```python
from build123d import *

# Parameters (mm, degrees)
F0_R     = 12.7
F1_DEPTH = 30.1625


with BuildPart() as f1:
    # F0 (on Front) → F1 (new body, symmetric)
    with BuildSketch(Plane.XZ):
        with BuildLine():
            Line((117.2464, 0), (22.352, 0))
            ThreePointArc((22.352, 0), (-15.805251, 15.805251), (0, -22.352))
            Line((0, -22.352), (194.2084, -22.352))
            Line((194.2084, -22.352), (194.2084, -7.874))
            ThreePointArc((194.2084, -7.874), (191.902159, -2.306241), (186.3344, 0))
            Line((186.3344, 0), (150.0886, 0))
            Line((150.0886, 0), (150.0886, 29.718))
            ThreePointArc((150.0886, 29.718), (148.600702, 33.310102), (145.0086, 34.798))
            Line((145.0086, 34.798), (131.0386, 34.798))
            ThreePointArc((131.0386, 34.798), (127.464415, 16.082358), (117.2464, 0))
        make_face()
        Circle(F0_R, mode=Mode.SUBTRACT)
    extrude(amount=F1_DEPTH, both=True)


solid = f1.part
```
Geometry check sheet. Reference: the model listing, model coordinates, mm. A direction names the side the tool comes from. Round coordinates to 2 decimals unless told otherwise and drop trailing zeros. Loops run counter-clockwise (first coordinate to the right, second up) from the corner with the lowest first, then second, coordinate; pieces in that order, holes last. Notation, with made-up numbers: (88.5, 2.25) - (117.5, 2.25) arc R17 ccw to (117.5, 22.25) - close; hole circle Ø4 at (-8.5, 86.5). An arc over 180 degrees is marked (long way). Use a Markdown table: item, result.
Q1. Go/stop test with flat-tipped pins: P1, Ø4, axis at x = 165.5, y = -19, coming from the +Z side; P2, Ø2, axis at y = 7, z = 29, coming from the -X side; P3, Ø12, axis at y = -2.5, z = 28.5, coming from the +X side. Record where each tip stops, or that it passes through.
Solutions:
| item | result |
|---|---|
| P1 | stops at z = 0 |
| P2 | stops at x = 130.58 |
| P3 | stops at x = 150.09 |
Q2. Cross-section at C-C on x = 93. Record the cut outline in (y, z).
Solutions:
| item | result |
|---|---|
| outline | (-30.16, -22.35) - (30.16, -22.35) - (30.16, 0) - (-30.16, 0) - close |
Q3. Material ranges on line 1 (Z direction, x = 0, y = -3); line 2 (X direction, y = 2, z = 4); line 3 (Z direction, x = 70, y = 26), recorded low to high.
Solutions:
| item | result |
|---|---|
| line 1 | z = -22.35 to -12.7, 12.7 to 22.35 |
| line 2 | x = -21.99 to -12.05, 12.05 to 21.99, 120.64 to 150.09 |
| line 3 | z = -22.35 to 0 |
Q4. Draft check along X on faces 4 (the cylindrical face through (191.963, -0.422, -2.368)), 5 (the flat face through (84, 30.162, -6)), 6 (the cylindrical face through (127.56, -0.42, 16.33)). Enter one of: released by +X, released by -X, zero draft, split by the parting line, or undercut.
Solutions:
| item | result |
|---|---|
| face 4 | released by +X |
| face 5 | zero draft |
| face 6 | undercut |
Q5. Cross-section at B-B on y = -17.5. Record the cut outline in (x, z).
Solutions:
| item | result |
|---|---|
| outline | (0, -22.35) - (194.21, -22.35) - (194.21, -7.87) arc R7.87 ccw to (186.33, 0) - (150.09, 0) - (150.09, 29.72) arc R5.08 ccw to (145.01, 34.8) - (131.04, 34.8) arc R50.8 cw to (117.25, 0) - (22.35, 0) arc R22.35 ccw (long way) to start; hole circle Ø25.4 at (0, 0) |
Q6. Access from +Z, -Z, +X, -X, +Y, -Y to the whole of each face (thin tool, end or side, straight path). Record for faces 1 (the flat face through (194.208, 0, -15)), 2 (the flat face through (150.089, 0, 15)), 3 (the flat face through (70, 0, 0)).
Solutions:
| item | result |
|---|---|
| face 1 | +Z, -Z, +X, +Y, -Y |
| face 2 | +Z, +X, +Y, -Y |
| face 3 | +Z, +Y, -Y |
Q7. Cross-section at A-A on z = 9.5. Record the cut outline in (x, y), plus the area to 3 significant figures.
Solutions:
| item | result |
|---|---|
| outline | (-20.23, -30.16) - (-8.43, -30.16) - (-8.43, 30.16) - (-20.23, 30.16) - close; (8.43, -30.16) - (20.23, -30.16) - (20.23, 30.16) - (8.43, 30.16) - close; (124.29, -30.16) - (150.09, -30.16) - (150.09, 30.16) - (124.29, 30.16) - close |
| area | 2,980 mm2 |
